from build123d import *

# Parameters (mm, degrees)
SKETCH1_W                    = 80
SKETCH1_H                    = 84
SKETCH1_R                    = 9.75
F_29_MM_EXTRUDE_DEPTH        = 29
SKETCH2_R                    = 28.5
F_7_MM_CUT_DEPTH             = 10
F_30R_FUNNEL_SLOPE_R         = 30
SKETCH3_R                    = 5.1
F_36_MM_CUT_SCREW_HEAD_DEPTH = 36
SKETCH5_R                    = 3.1
F_7_8MM_BORE_DEPTH           = 95.89467846
F_3R_PIG_HOLE_R              = 3
F_2R_CORNERS_R               = 2
F_0_5R_BOLTS_R               = 0.5


with BuildPart() as part:
    # Sketch1 → 29 mm extrude (new body)
    with BuildSketch(Plane(origin=(0, 0, 0), x_dir=(0, 1, 0), z_dir=(0, 0, 1))):
        Rectangle(SKETCH1_W, SKETCH1_H)
        with Locations(Location((0, 0, 0), (0, 0, 90))):
            Circle(SKETCH1_R, mode=Mode.SUBTRACT)
    extrude(amount=F_29_MM_EXTRUDE_DEPTH)

    # Sketch2 → 7 mm cut (cut)
    with BuildSketch(Plane(origin=(0, 0, 0), x_dir=(1, 0, 0), z_dir=(0, 0, -1))):
        with Locations(Location((0, 0, 0), (0, 0, 180))):
            Circle(SKETCH2_R)
    extrude(amount=-F_7_MM_CUT_DEPTH, mode=Mode.SUBTRACT)

    # 30R funnel slope
    # the kernel refuses this fillet: 30 mm, written as the material it takes off along each edge
    with BuildSketch(Plane(origin=(0, 0, 29), x_dir=(-1, 0, 0), z_dir=(0, 1, 0))) as f_30r_funnel_slope_piece_1:
        with BuildLine():
            CenterArc((37.660571474, -30), F_30R_FUNNEL_SLOPE_R, 90, 68.489811733)
            Line((9.75, -19), (9.191788571, -18.78))
            ThreePointArc((9.191788571, -18.78), (9.15, -9.5), (9.15, 0))
            Line((9.15, 0), (9.75, 0.6))
            Line((9.75, 0.6), (37.660571474, 0.6))
            Line((37.660571474, 0.6), (37.660571474, 0))
        make_face()
    revolve(axis=Axis((0, 0, 29), (0, 0, 1)), mode=Mode.SUBTRACT)

    # Sketch3 → 36 mm cut screw head (cut)
    with BuildSketch(Plane(origin=(0, 40, 0), x_dir=(-1, 0, 0), z_dir=(0, 1, 0))):
        with Locations((-35.025, 14.5)):
            Circle(SKETCH3_R)
        with Locations((35.025, 14.5)):
            Circle(SKETCH3_R)
    extrude(amount=-F_36_MM_CUT_SCREW_HEAD_DEPTH, mode=Mode.SUBTRACT)

    # Sketch5 → 7.8mm bore (cut, through all)
    with BuildSketch(Plane(origin=(0, 40, 0), x_dir=(-1, 0, 0), z_dir=(0, 1, 0))):
        with Locations((-35.025, 14.5)):
            Circle(SKETCH5_R)
    f_7_8mm_bore = extrude(amount=-F_7_8MM_BORE_DEPTH, mode=Mode.SUBTRACT)

    # 3R pig hole
    f_3r_pig_hole_edges = [part.edges().sort_by_distance(p)[0] for p in [
        (28.5, 0, 10),
    ]]
    fillet(f_3r_pig_hole_edges, radius=F_3R_PIG_HOLE_R)

    # 2R corners
    # the kernel refuses this fillet: 2 mm, written as the material it takes off along each edge
    with BuildSketch(Plane(origin=(42, 40, -5), x_dir=(0, -1, 0), z_dir=(0, 0, 1)), Plane(origin=(-42, 40, -5), x_dir=(1, 0, 0), z_dir=(0, 0, 1))) as f_2r_corners_piece_1:
        with BuildLine():
            CenterArc((F_2R_CORNERS_R, -F_2R_CORNERS_R), F_2R_CORNERS_R, 90, 90)
            Line((0, -F_2R_CORNERS_R), (0, 0))
            Line((0, 0), (F_2R_CORNERS_R, 0))
        make_face()
    extrude(amount=39, mode=Mode.SUBTRACT)
    with BuildSketch(Plane(origin=(42, -40, -5), x_dir=(0, 1, 0), z_dir=(0, 0, 1)), Plane(origin=(-42, -40, -5), x_dir=(1, 0, 0), z_dir=(0, 0, 1))) as f_2r_corners_piece_2:
        with BuildLine():
            CenterArc((F_2R_CORNERS_R, F_2R_CORNERS_R), F_2R_CORNERS_R, 180, 90)
            Line((0, F_2R_CORNERS_R), (0, 0))
            Line((0, 0), (F_2R_CORNERS_R, 0))
        make_face()
    extrude(amount=39, mode=Mode.SUBTRACT)

    # 0.5R bolts
    f_0_5r_bolts_edges = [part.edges().sort_by_distance(p)[0] for p in [
        (-29.925, 40, 14.5),
        (34.46042051, 40, 19.568653667),
        (-40.093653599, 39.997806015, 15.064580313),
        (40.125, 39.996089928, 14.5),
    ]]
    fillet(f_0_5r_bolts_edges, radius=F_0_5R_BOLTS_R)

    # Mirror1: 7.8mm bore across plane
    add(f_7_8mm_bore.mirror(Plane(origin=(0, 0, 0), x_dir=(0, 0, 1), z_dir=(1, 0, 0))), mode=Mode.SUBTRACT)


solid = part.part
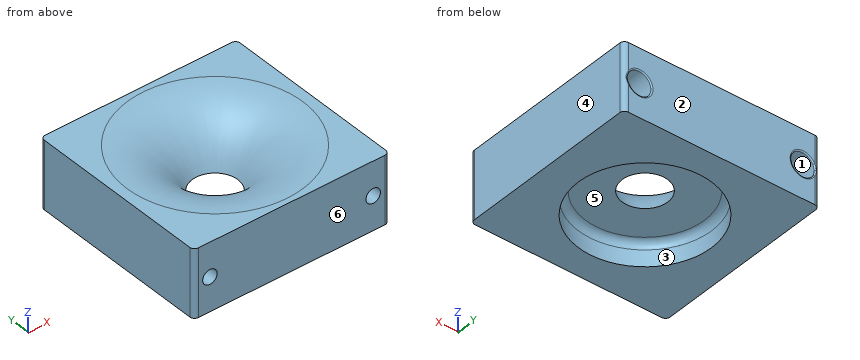
Could you check a few things on this model? Use its own coordinates, in mm. Face numbers are marked on the shaded views. A direction names the side the tool comes from. Give positions to 0.01 mm unless a question says otherwise; leave off trailing zeros. Order: outer loops, then holes, each group sorted by start corner. A loop starts at its lowest first (then second) coordinate and runs counter-clockwise, first axis right, second up.
1. Will these pins go through, and if not, where does the flat tip stop? P1, Ø6, axis at x = 8, y = -1, coming from the -Z side; P2, Ø8, axis at x = 37.5, z = 16, coming from the +Y side; P3, Ø8, axis at x = -35.025, z = 14.5, coming from the +Y side; P4, Ø10, axis at x = 21, y = 5, coming from the -Z side.
2. Suppose I cut it at B-B (x = 0). List the corners of the cut face in (y, z) for me, plus the area to 3 significant figures.
3. I need wall thicknesses on L1, parallel to X at y = 11.5, z = 17; L2, parallel to Y at x = 0, z = 3; L3, parallel to X at y = 14, z = 11.5. Which ranges of each line are inside material? Lowest first, please.
4. For the marked faces 1 and 2, which set-ups out of +Z, -Z, +X, -X, +Y, -Y let a thin tool reach every point of the face, with its end or its side?
5. We'd pull the mould along Y, two halves only. Please class the marked faces 3, 4, 5 and 6: pulls with the +Y half, pulls with the -Y half, needs draft (parallel to the pull), parting line crosses it, or undercut.
6. Suppose I cut it at A-A (y = 0). List the corners of the cut face in (x, z) for me (3 decimals).
7. Suppose I cut it at C-C (y = 21). Give the number of separate pieces and of enclosed holes in the cut face, plus the area to 3 significant figures.
Solved:
1. P1: stops at z = 10
1. P2: stops at y = 40
1. P3: stops at y = 4
1. P4: stops at z = 9.8
2. outline: (-40, 0) - (-28.5, 0) - (-28.5, 7) arc R3 cw to (-25.5, 10) - (-9.75, 10) arc R30 ccw to (-37.66, 29) - (-40, 29) - close; (9.75, 10) - (25.5, 10) arc R3 cw to (28.5, 7) - (28.5, 0) - (40, 0) - (40, 29) - (37.66, 29) arc R30 ccw to start
2. area: 1,090 mm2
3. L1: x = -42 to -39.47, -30.58 to -7.37, 7.37 to 30.58, 39.47 to 42
3. L2: y = -40 to -28.5, 28.5 to 40
3. L3: x = -42 to -39.15, -30.9 to 30.9, 39.15 to 42
4. face 1: +Y
4. face 2: +Z, -Z, +X, -X, +Y
5. face 3: undercut
5. face 4: needs draft
5. face 5: undercut
5. face 6: pulls with the -Y half
6. outline: (-42, 0) - (-28.5, 0) - (-28.5, 7) arc R3 cw to (-25.5, 10) - (-9.75, 10) arc R30 ccw to (-37.661, 29) - (-42, 29) - close; (9.75, 10) - (25.5, 10) arc R3 cw to (28.5, 7) - (28.5, 0) - (42, 0) - (42, 29) - (37.661, 29) arc R30 ccw to start; hole circle Ø6.2 at (-35.025, 14.5); hole circle Ø6.2 at (35.025, 14.5)
7. separate pieces: 1
7. enclosed holes: 2
7. area: 1,740 mm2
